Check sheet for the modelled part. Datum: model origin and axes. Units: mm. Face numbers are marked on the shaded views. A direction names the side the tool comes from. Coordinates: 2 decimals unless noted, no trailing zeros. Loops run counter-clockwise (first coordinate to the right, second up) from the corner with the lowest first, then second, coordinate; pieces in that order, holes last. Notation, with made-up numbers: (66.25, 79) - (93.25, 79) arc R22 cw to (93.25, 115) - close; hole circle Ø11 at (-18.75, 23). An arc over 180 degrees is marked (long way). Write each question's results on one line, items separated by ' | '. Start each with the question number.
1. Draft check along Z on the marked faces 3, 4 and 5. Enter one of: released by +Z, released by -Z, zero draft, split by the parting line, or undercut.
2. Cross-section at A-A (x = -1.75). Record the cut outline in (y, z).
3. Thickness scan on line 1 (Y direction, x = -2.5, z = 4.75); line 2 (X direction, y = -0.25, z = 2.5); line 3 (X direction, y = -3.75, z = 4.25). Record the ranges inside material, lowest first. Write a range as [from, to].
4. Cross-section at C-C (z = 2.7). Record the cut outline in (x, y).
5. Tool access check on the marked faces 1 and 2. Record the directions out of +Z, -Z, +X, -X, +Y, -Y that give a thin tool (end or side, any length) a straight path to the whole face; none if there is none.
6. Gauge pin test, flat ends, axial feed: P1, Ø1, axis at x = 1, y = 1.5, coming from the +Z side; P2, Ø2, axis at x = -1.5, y = -2.5, coming from the -Z side; P3, Ø3, axis at y = -2, z = -6, coming from the -X side. Record the tip position at first contact, or that the pin passes through.
7. Cross-section at D-D (z = -1). Record the cut outline in (x, y), and give its area (3 significant figures).
```python
from build123d import *

# Parameters (mm, degrees)
SKETCH_R     = 7.5
PAD_DEPTH    = 2
SKETCH001_R  = 4.75
PAD001_DEPTH = 4
SKETCH002_R  = 2.05
POCKET_DEPTH = 6
PAD002_DEPTH = 2
PAD003_DEPTH = 2


with BuildPart() as part:
    # Sketch → Pad (new body)
    with BuildSketch(Plane.XZ):
        Circle(SKETCH_R)
    extrude(amount=PAD_DEPTH)

    # Sketch001 (on Face3 of Pad) → Pad001 (join)
    with BuildSketch(Plane.XZ.offset(2)):
        Circle(SKETCH001_R)
    extrude(amount=PAD001_DEPTH)

    # Sketch002 (on Face5 of Pad001) → Pocket (cut)
    with BuildSketch(Plane.XZ.offset(6)):
        with Locations((0, 2.7)):
            Circle(SKETCH002_R)
    extrude(amount=-POCKET_DEPTH, mode=Mode.SUBTRACT)

    # Sketch003 (on Face2 of Pocket) → Pad002 (join)
    with BuildSketch(Plane(origin=(0, 0, 0), x_dir=(1, 0, 0), z_dir=(0, 1, 0))):
        with BuildLine():
            Line((-4.069398, 6.3), (4.069398, 6.3))
            ThreePointArc((4.069398, 6.3), (0, 9.3), (-4.069398, 6.3))
        make_face()
    extrude(amount=PAD002_DEPTH)

    # Pad002 Face3 → Pad003 (add)
    with BuildSketch(Plane(origin=(0, 0, -7.992176), x_dir=(-1, 0, 0), z_dir=(0, -1, 0))):
        with BuildLine():
            ThreePointArc((4.069398, -1.692176), (0, 1.307824), (-4.069398, -1.692176))
            ThreePointArc((-4.069398, -1.692176), (0, -0.492176), (4.069398, -1.692176))
        make_face()
    extrude(amount=PAD003_DEPTH)


solid = part.part
```
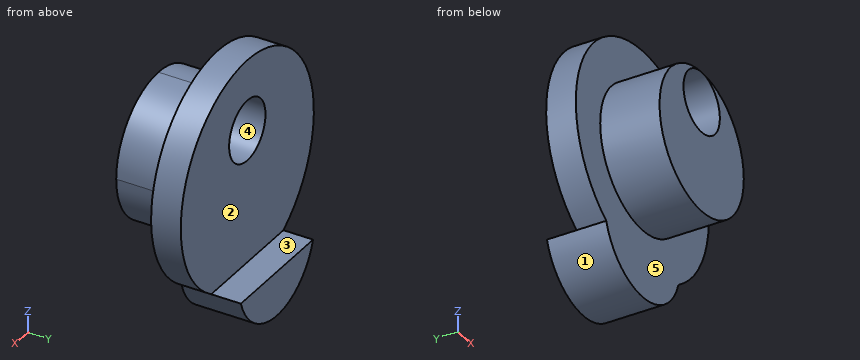
Established:
1) face 3: released by +Z | face 4: undercut | face 5: zero draft
2) outline: (-6, -4.42) - (-2, -4.42) - (-2, -8.92) - (2, -8.92) - (2, -6.3) - (0, -6.3) - (0, 1.63) - (-6, 1.63) - close; (-6, 3.77) - (0, 3.77) - (0, 7.29) - (-2, 7.29) - (-2, 4.42) - (-6, 4.42) - close
3) line 1: [-2, 0] | line 2: [-7.07, -2.04], [2.04, 7.07] | line 3: [-2.12, -1.34], [1.34, 2.12]
4) outline: (-7, -2) - (-3.91, -2) - (-3.91, -6) - (-2.05, -6) - (-2.05, 0) - (-7, 0) - close; (2.05, -6) - (3.91, -6) - (3.91, -2) - (7, -2) - (7, 0) - (2.05, 0) - close
5) face 1: -Z, +Y, -Y | face 2: +Z, +X, -X, +Y
6) P1: z = -6.3 | P2: z = -9.25 | P3: x = -6
7) outline: (-7.43, -2) - (-4.64, -2) - (-4.64, -6) - (4.64, -6) - (4.64, -2) - (7.43, -2) - (7.43, 0) - (-7.43, 0) - close | area: 66.9 mm^2
